CAD build for the part. Positions are in the model's coordinates, mm. Give positions to 0.01 mm unless a question says otherwise; leave off trailing zeros. Order: outer loops, then holes, each group sorted by start corner. A loop starts at its lowest first (then second) coordinate and runs counter-clockwise, first axis right, second up.
from build123d import *

# Parameters (mm, degrees)
SKETCH_1_W          = 20
SKETCH_1_H          = 31
EXTRUDE_1_DEPTH     = 10.7
SKETCH_2_R          = 1.25
CUT_EXTRUDE_1_DEPTH = 40.7
CHAMFER_1_SIZE      = 8
SKETCH_3_R          = 2
EXTRUDE_2_DEPTH     = 0.5
FILLET_1_R          = 3


with BuildPart() as part:
    # 草图1 → 凸台-拉伸1 (new body)
    with BuildSketch(Plane(origin=(0, 0, 0), x_dir=(1, 0, 0), z_dir=(0, 1, 0))):
        Rectangle(SKETCH_1_W, SKETCH_1_H)
    extrude(amount=EXTRUDE_1_DEPTH)

    # 草图2 → 切除-拉伸1 (cut)
    with BuildSketch(Plane(origin=(0, 10.7, 0), x_dir=(1, 0, 0), z_dir=(0, 1, 0))):
        with Locations(Location((-7, 12.7, 0), (0, 0, 270))):
            Circle(SKETCH_2_R)
        with Locations(Location((-7, -12.7, 0), (0, 0, 90))):
            Circle(SKETCH_2_R)
    extrude(amount=-CUT_EXTRUDE_1_DEPTH, mode=Mode.SUBTRACT)

    # 倒角1
    chamfer_1_edges = [part.edges().sort_by_distance(p)[0] for p in [
        (10, 5.35, 15.5),
    ]]
    chamfer(chamfer_1_edges, length=CHAMFER_1_SIZE)

    # 草图3 → 凸台-拉伸2 (add)
    with BuildSketch(Plane(origin=(8.75, 0, 8.75), x_dir=(0.7071067811865485, 0, -0.7071067811865466), z_dir=(0.7071067811865466, 0, 0.7071067811865485))):
        with Locations((-3.889087297, 5.35)):
            Circle(SKETCH_3_R)
    extrude(amount=EXTRUDE_2_DEPTH)

    # 圆角1
    fillet_1_edges = [part.edges().sort_by_distance(p)[0] for p in [
        (-10, 5.35, -15.5),
        (-10, 5.35, 15.5),
    ]]
    fillet(fillet_1_edges, radius=FILLET_1_R)


solid = part.part
1. Saw through at A-A on y = 9. Give the cut face in (x, z).
2. Saw through at B-B on x = 3.5. Give the cut face in (y, z).
3. Saw through at C-C on y = 7. Give the cut face in (x, z), plus the area to 3 significant figures.
4. Mould opens along Z. For faces 1 (the cylindrical face through (-5.891, 5.425, 12.123)), 2 (the flat face through (10, 5, -4)), 3 (the cylindrical face through (-7.479, 5.425, -11.545)), 4 (the flat face through (6.334, 5.378, 11.873)) say: released by +Z, released by -Z, zero draft, split by the parting line, or undercut.
5. Pin check, flat tip, straight feed: P1, Ø2, axis at x = -7, z = 12.7, coming from the -Y side. Stop position of the tip, or through.
6. Saw through at D-D on z = 14.5. Give the cut face in (x, y).
7. Wall check: line 1 (Z direction, x = -8, y = 4.75); line 2 (Z direction, x = -6.25, y = 9.75); line 3 (X direction, y = 4.25, z = -12.7). Give the ranges that are in metal, low to high.
Reported:
1. outline: (-10, -12.5) arc R3 ccw to (-7, -15.5) - (10, -15.5) - (10, 7.5) - (2, 15.5) - (-7, 15.5) arc R3 ccw to (-10, 12.5) - close; hole circle Ø2.5 at (-7, -12.7); hole circle Ø2.5 at (-7, 12.7)
2. outline: (0, -15.5) - (10.7, -15.5) - (10.7, 14) - (0, 14) - close
3. outline: (-10, -12.5) arc R3 ccw to (-7, -15.5) - (10, -15.5) - (10, 7.5) - (6.8, 10.7) - (7.15, 11.05) - (5.55, 12.65) - (5.2, 12.3) - (2, 15.5) - (-7, 15.5) arc R3 ccw to (-10, 12.5) - close; hole circle Ø2.5 at (-7, -12.7); hole circle Ø2.5 at (-7, 12.7)
3. area: 575 mm2
4. face 1: undercut
4. face 2: zero draft
4. face 3: undercut
4. face 4: released by +Z
5. P1: passes through
6. outline: (-9.24, 0) - (3, 0) - (3, 10.7) - (-9.24, 10.7) - close
7. line 1: z = -15.33 to -13.45, -11.95 to 11.95, 13.45 to 15.33
7. line 2: z = -15.5 to -13.7, -11.7 to 11.7, 13.7 to 15.5
7. line 3: x = -9.99 to -8.25, -5.75 to 10
